Verification items for the finished model (mm, model axes). Round coordinates to 2 decimals unless told otherwise and drop trailing zeros. Write each loop counter-clockwise with the first axis right and the second up, starting at its lowest first coordinate (ties: lowest second). Pieces come first, ordered by that corner, then holes. Notation, with made-up numbers: M -17,55.5 L 8,55.5 A23 cw 8,81.5 Z; hole C 18,73 d2. An arc over 180 degrees is marked long. Answer in a Markdown table with one row per item. Add a question column.
1. Material ranges on probe 1 along Z at (x, y) = (-35, -69.5); probe 2 along Z at (x, y) = (-25, -88); probe 3 along Y at (x, z) = (30.5, -60), recorded low to high.
2. Sectioned sample at A-A on x = 60. Record the cut outline in (y, z).
3. Go/stop test with flat-tipped pins: pin 1 Ø3 at (x, z) = (13, -47.5) entering from -Y; pin 2 Ø1.5 at (x, z) = (70.5, -8.5) entering from -Y. Record where each tip stops, or that it passes through.
```python
from build123d import *

# Parameters (mm, degrees)
F0_W     = 203.2
F0_H     = 203.2
F1_DEPTH = 101.6
F2_R     = 101.6
F3_DEPTH = 203.201
F4_SIZE  = 5.08


with BuildPart() as f1:
    # F0 (on Right) → F1 (new body, symmetric)
    with BuildSketch(Plane.YZ):
        Rectangle(F0_W, F0_H)
    extrude(amount=F1_DEPTH, both=True)

    # F2 (on face) → F3 (cut, through all)
    with BuildSketch(Plane.YZ.offset(101.6)):
        with Locations((-101.6, -101.6)):
            Circle(F2_R)
    extrude(amount=-F3_DEPTH, mode=Mode.SUBTRACT)

    # F4
    f4_edges = [f1.edges().sort_by_distance(p)[0] for p in [
        (101.6, 0, 101.6),
        (101.6, 101.6, 0),
        (101.6, 50.8, -101.6),
        (101.6, -29.757951, -29.757951),
        (101.6, -101.6, 50.8),
        (-101.6, 0, 101.6),
        (0, -101.6, 101.6),
        (0, 101.6, 101.6),
    ]]
    chamfer(f4_edges, length=F4_SIZE)


solid = f1.part
```
Geometry check:
| question | item | result |
|---|---|---|
| 1 | probe 1 | z = -5.2 to 101.6 |
| 1 | probe 2 | z = -0.91 to 101.6 |
| 1 | probe 3 | y = -8.91 to 101.6 |
| 2 | outline | M -101.6,0 A101.6 cw 0,-101.6 L 101.6,-101.6 L 101.6,96.52 L 96.52,101.6 L -96.52,101.6 L -101.6,96.52 Z |
| 3 | pin 1 | stops at y = -16.56 |
| 3 | pin 2 | stops at y = -62.68 |
